Geometry: final body of the model. Coordinates: model frame, mm. A direction names the side the tool comes from. Round coordinates to 2 decimals unless told otherwise and drop trailing zeros. Loops run counter-clockwise (first coordinate to the right, second up) from the corner with the lowest first, then second, coordinate; pieces in that order, holes last. Notation, with made-up numbers: (-2, 40) -> (42, 40) arc R12 ccw to (42, 48) -> close; hole circle Ø9 at (80, -13). An arc over 180 degrees is marked (long way). Answer in a Markdown table with one row per item.
Autodesk Inventor part; units mm, degrees
ref_plane "YZ Plane" through (0, 0, 0) normal (1, 0, 0) x (0, 1, 0)
ref_plane "XZ Plane" through (0, 0, 0) normal (0, 1, 0) x (-1, 0, 0)
ref_plane "XY Plane" through (0, 0, 0) normal (0, 0, 1) x (1, 0, 0)
sketch "Skizze1" plane through (0, 0, 0) normal (0, 1, 0) x (-1, 0, 0)
  line L0 (-6.5, -8.75) -> (6.5, -8.75)
  line L1 (6.5, -8.75) -> (6.5, 8.75)
  line L2 (6.5, 8.75) -> (-6.5, 8.75)
  line L3 (-6.5, 8.75) -> (-6.5, -8.75)
  line L4 (-6.5, -8.75) -> (6.5, 8.75) construction
  line L5 (6.5, -8.75) -> (-6.5, 8.75) construction
  point P0 (0, 0)
  dimension "d0" = 13
  dimension "d1" = 17.5
extrude "Extrusion1" add sketch "Skizze1" along normal blind 5.5
sketch "Skizze2" plane through (0, 5.5, 0) normal (0, 1, 0) x (1, 0, 0)
  line L0 (-6.5, 8.75) -> (-6.5, -8.75)
  line L1 (-6.5, -8.75) -> (6.5, -8.75)
  line L2 (6.5, -8.75) -> (6.5, 8.75)
  line L3 (6.5, 8.75) -> (-6.5, 8.75)
  line L4 (3.75, -4.4349) -> (-3.75, -4.4349)
  line L5 (-3.75, -4.4349) -> (-3.75, -8.4349)
  line L6 (-3.75, -8.4349) -> (3.75, -8.4349)
  line L7 (3.75, -8.4349) -> (3.75, -4.4349)
  line L8 (3.75, -4.4349) -> (-3.75, -8.4349) construction
  line L9 (-3.75, -4.4349) -> (3.75, -8.4349) construction
  point P0 (0, 0)
  point P1 (0, -6.4349)
  dimension "d4" = 7.5
  dimension "d5" = 4
extrude "Extrusion2" cut sketch "Skizze2" against normal blind 1 contours L7 L6 L5 L4
sketch "Skizze3" plane through (0, 5.5, 0) normal (0, 1, 0) x (1, 0, 0)
  line L0 (-6.5, 8.75) -> (-6.5, -8.75)
  line L1 (3.75, -8.4349) -> (-3.75, -8.4349)
  line L2 (-3.75, -8.4349) -> (-3.75, -4.4349)
  line L3 (-3.75, -4.4349) -> (3.75, -4.4349)
  line L4 (3.75, -4.4349) -> (3.75, -8.4349)
  line L5 (-6.5, 8.75) -> (-6.5, -8.75)
  line L6 (-6.5, -8.75) -> (6.5, -8.75)
  line L7 (6.5, -8.75) -> (6.5, 8.75)
  line L8 (6.5, 8.75) -> (-6.5, 8.75)
  line L9 (6.5, -8.75) -> (6.5, 8.75)
  line L10 (-6.5, -8.75) -> (6.5, -8.75)
  line L11 (6.5, -8.75) -> (6.5, -2.25)
  line L12 (6.5, -2.25) -> (-6.5, -2.25)
  line L13 (-6.5, -2.25) -> (-6.5, -8.75)
  point P0 (0, 0)
  dimension "d8" = 6.5
extrude "Extrusion3" cut sketch "Skizze3" against normal blind 0.1 contours L12 L7 L6 L0
sketch "Skizze4" plane through (6.5, 0, -8.75) normal (0, 0, -1) x (-1, 0, 0)
  line L0 (0, 0) -> (13, 0)
  line L1 (13, 0) -> (13, 5.5)
  line L2 (0, 5.5) -> (13, 5.5)
  line L3 (0, 0) -> (0, 5.5)
  line L4 (10.15, 4.75) -> (2.85, 4.75)
  line L5 (2.85, 4.75) -> (2.85, 0.75)
  line L6 (2.85, 0.75) -> (10.15, 0.75)
  line L7 (10.15, 0.75) -> (10.15, 4.75)
  line L8 (10.15, 4.75) -> (2.85, 0.75) construction
  line L9 (2.85, 4.75) -> (10.15, 0.75) construction
  point P0 (6.5, 0)
  point P1 (6.5, 2.75)
  dimension "d11" = 7.3
  dimension "d12" = 4
extrude "Extrusion4" cut sketch "Skizze4" against normal blind 0.1 contours L7 L6 L5 L4
properties part number "00_HuaweiP30_Telelens"
Item 1: Reachability of faces 4 (the face through (0, 5, 8.435)), 5 (the face through (0, 5.5, -3)), 6 (the face through (0, 5.4, 4)) from +Z, -Z, +X, -X, +Y, -Y: full face, straight path, thin tool, end or side. Return the list, or none.
Answer:
| item | result |
|---|---|
| face 4 | +Y |
| face 5 | +Z, -Z, +X, -X, +Y |
| face 6 | +Z, +X, -X, +Y |
Item 2: Cut plane B-B (x = -2). Output: boundary loops of the cut face in (y, z).
Answer:
| item | result |
|---|---|
| outline | (0, -8.75) -> (0.75, -8.75) -> (0.75, -8.65) -> (4.75, -8.65) -> (4.75, -8.75) -> (5.5, -8.75) -> (5.5, 2.25) -> (5.4, 2.25) -> (5.4, 4.43) -> (4.5, 4.43) -> (4.5, 8.43) -> (5.4, 8.43) -> (5.4, 8.75) -> (0, 8.75) -> close |
Item 3: Line query: probe 1 along Z at (x, y) = (0, 5); probe 2 along Z at (x, y) = (3.5, 0.95); probe 3 along Y at (x, z) = (4.5, 7). Output: solid intervals per line, ascending. Write a range as [from, to].
Answer:
| item | result |
|---|---|
| probe 1 | z = [-8.75, 4.43], [8.43, 8.75] |
| probe 2 | z = [-8.65, 8.75] |
| probe 3 | y = [0, 5.4] |
Item 4: Cut plane A-A (y = 5.15). Output: boundary loops of the cut face in (x, z).
Answer:
| item | result |
|---|---|
| outline | (-6.5, -8.75) -> (6.5, -8.75) -> (6.5, 8.75) -> (-6.5, 8.75) -> close; hole (-3.75, 4.43) -> (3.75, 4.43) -> (3.75, 8.43) -> (-3.75, 8.43) -> close |
Item 5: Pin query (flat end, axial travel): pin 1 Ø1.2 at (x, z) = (1, 6) entering from +Y. Return the tip coordinate at first contact, or that it passes through.
Answer:
| item | result |
|---|---|
| pin 1 | stops at y = 4.5 |
Item 6: Draft query along Z for faces 1 (the face through (0, 0, 0)), 2 (the face through (0, 3, -8.65)), 3 (the face through (0, 4.5, 6)). Return one class per face: pulls with the +Z half, pulls with the -Z half, needs draft (parallel to the pull), parting line crosses it, or undercut.
Answer:
| item | result |
|---|---|
| face 1 | needs draft |
| face 2 | pulls with the -Z half |
| face 3 | undercut |
Item 7: Cut plane C-C (z = 2.75). Output: boundary loops of the cut face in (x, y).
Answer:
| item | result |
|---|---|
| outline | (-6.5, 0) -> (6.5, 0) -> (6.5, 5.4) -> (-6.5, 5.4) -> close |
